Work out the finished part from the listing and answer in its coordinate system (mm). Face numbers are marked on the shaded views. A direction names the side the tool comes from. Give positions to 0.01 mm unless a question says otherwise; leave off trailing zeros. Order: outer loops, then holes, each group sorted by start corner. A loop starts at its lowest first (then second) coordinate and runs counter-clockwise, first axis right, second up.
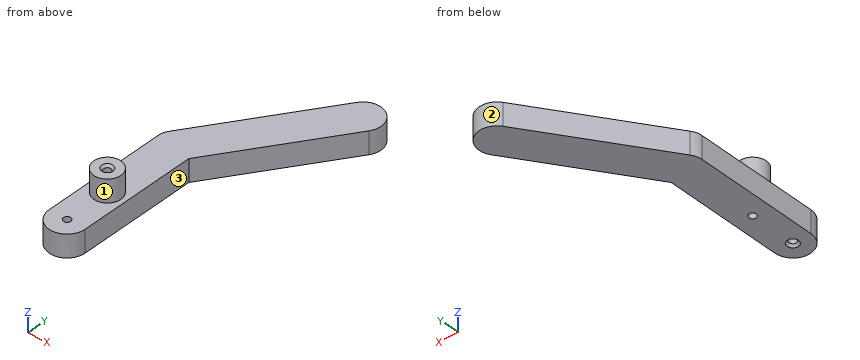
```python
from build123d import *

# Parameters (mm, degrees)
F1_DEPTH       = 6.35
F2_R           = 3.81
F3_DEPTH       = 12.7
F5_D           = 2.032
F5_CSINK_D     = 3.175
F5_CSINK_ANGLE = 82
F6_D           = 2.032
F6_CSINK_D     = 3.175
F6_CSINK_ANGLE = 82


with BuildPart() as f1:
    # F0 (on Top) → F1 (new body)
    with BuildSketch(Plane.XY):
        with BuildLine():
            ThreePointArc((-5.08, 12.7), (-3.5921024484, 9.1078975516), (0, 7.62))
            Line((0, 7.62), (0, 12.7))
            Line((0, 12.7), (0, 17.78))
            ThreePointArc((0, 17.78), (-3.5921024484, 16.2921024484), (-5.08, 12.7))
        make_face()
        with BuildLine():
            Line((0, 12.7), (0, 7.62))
            ThreePointArc((0, 7.62), (3.5921024484, 9.1078975516), (5.08, 12.7))
            ThreePointArc((5.08, 12.7), (3.5921024484, 16.2921024484), (0, 17.78))
            Line((0, 17.78), (0, 12.7))
        make_face()
        with BuildLine():
            ThreePointArc((5.08, 12.7), (3.5921024484, 9.1078975516), (0, 7.62))
            ThreePointArc((0, 7.62), (-3.5921024484, 9.1078975516), (-5.08, 12.7))
            Line((-5.08, 12.7), (-5.08, 0))
            ThreePointArc((-5.08, 0), (0, -5.08), (5.08, 0))
            Line((5.08, 0), (5.08, 12.7))
        make_face()
        with BuildLine():
            ThreePointArc((0, 17.78), (3.5921024484, 16.2921024484), (5.08, 12.7))
            Line((5.08, 12.7), (5.08, 32.7368881382))
            Line((5.08, 32.7368881382), (4.2115108686, 31.4493000504))
            ThreePointArc((4.2115108686, 31.4493000504), (2.384915539, 29.8046262283), (0, 29.21))
            Line((0, 29.21), (0, 17.78))
        make_face()
        with BuildLine():
            Line((-5.08, 34.29), (-5.08, 12.7))
            ThreePointArc((-5.08, 12.7), (-3.5921024484, 16.2921024484), (0, 17.78))
            Line((0, 17.78), (0, 29.21))
            ThreePointArc((0, 29.21), (-3.5921024484, 30.6978975516), (-5.08, 34.29))
        make_face()
        with BuildLine():
            Line((5.08, 34.29), (5.08, 32.7368881382))
            Line((5.08, 32.7368881382), (26.9371104656, 65.141386999))
            ThreePointArc((26.9371104656, 65.141386999), (25.5662995467, 72.1935978172), (18.5140887285, 70.8227868983))
            Line((18.5140887285, 70.8227868983), (-4.2115108686, 37.1306999496))
            ThreePointArc((-4.2115108686, 37.1306999496), (-0.9693096965, 39.2766660919), (2.8406999496, 38.5015108686))
            ThreePointArc((2.8406999496, 38.5015108686), (4.4853737717, 36.674915539), (5.08, 34.29))
        make_face()
        with BuildLine():
            Line((4.2115108686, 31.4493000504), (5.08, 32.7368881382))
            Line((5.08, 32.7368881382), (5.08, 34.29))
            ThreePointArc((5.08, 34.29), (4.4853737717, 36.674915539), (2.8406999496, 38.5015108686))
            Line((2.8406999496, 38.5015108686), (0, 34.29))
            Line((0, 34.29), (0, 29.21))
            ThreePointArc((0, 29.21), (2.384915539, 29.8046262283), (4.2115108686, 31.4493000504))
        make_face()
        with BuildLine():
            ThreePointArc((-4.2115108686, 37.1306999496), (-4.8580281603, 35.77524826), (-5.08, 34.29))
            ThreePointArc((-5.08, 34.29), (-3.5921024484, 30.6978975516), (0, 29.21))
            Line((0, 29.21), (0, 34.29))
            Line((0, 34.29), (2.8406999496, 38.5015108686))
            ThreePointArc((2.8406999496, 38.5015108686), (-0.9693096965, 39.2766660919), (-4.2115108686, 37.1306999496))
        make_face()
    extrude(amount=F1_DEPTH)

    # F2 (on Top) → F3 (join)
    with BuildSketch(Plane.XY):
        with Locations((0, 12.7)):
            Circle(F2_R)
    extrude(amount=F3_DEPTH)

    # F5 (through all)
    with Locations(Plane.XY.offset(12.7)):
        with Locations((0, 12.7)):
            CounterSinkHole(F5_D / 2, F5_CSINK_D / 2, counter_sink_angle=F5_CSINK_ANGLE)

    # F6 (through all)
    with Locations(Plane(origin=(0, 0, 0), x_dir=(1, 0, 0), z_dir=(0, 0, -1))):
        with Locations((0, 0)):
            CounterSinkHole(F6_D / 2, F6_CSINK_D / 2, counter_sink_angle=F6_CSINK_ANGLE)


solid = f1.part
```
1. Given P1, Ø7, axis at y = 23, z = 4, coming from the +X side; P2, Ø3, axis at y = 58.5, z = 2, coming from the +X side; P3, Ø2.5, axis at x = 0, y = 0, coming from the -Z side, each flat-ended and moving along its own axis, determine where each tip first touches the part or whether it passes through.
Findings below:
P1: stops at x = 5.08
P2: stops at x = 23.47
P3: stops at z = 0.39
2. The part is cut by section A-A (y = 12.7). Write down the section's boundary in (x, z).
Findings below:
outline: (-5.08, 0) - (-1.02, 0) - (-1.02, 12.04) - (-1.59, 12.7) - (-3.81, 12.7) - (-3.81, 6.35) - (-5.08, 6.35) - close; (1.02, 0) - (5.08, 0) - (5.08, 6.35) - (3.81, 6.35) - (3.81, 12.7) - (1.59, 12.7) - (1.02, 12.04) - close
3. Which of the six approach directions +Z, -Z, +X, -X, +Y, -Y give full straight-line access (tool end or side, diameter ignored) to the marked faces 1, 2 and 3?
Findings below:
face 1: +Z
face 2: +Z, -Z
face 3: +Z, -Z, +X, -Y
4. The part is cut by section C-C (z = 2.5). Write down the section's boundary in (x, y).
Findings below:
outline: (-5.08, 0) arc R5.08 ccw to (5.08, 0) - (5.08, 32.74) - (26.94, 65.14) arc R5.08 ccw to (18.51, 70.82) - (-4.21, 37.13) arc R5.08 ccw to (-5.08, 34.29) - close; hole circle Ø2.03 at (0, 0); hole circle Ø2.03 at (0, 12.7)
5. The part is cut by section B-B (x = 0). Write down the section's boundary in (y, z), then the cut area to 3 significant figures.
Findings below:
outline: (-5.08, 0) - (-1.59, 0) - (-1.02, 0.66) - (-1.02, 6.35) - (-5.08, 6.35) - close; (1.02, 0.66) - (1.59, 0) - (11.68, 0) - (11.68, 12.04) - (11.11, 12.7) - (8.89, 12.7) - (8.89, 6.35) - (1.02, 6.35) - close; (13.72, 0) - (43.37, 0) - (43.37, 6.35) - (16.51, 6.35) - (16.51, 12.7) - (14.29, 12.7) - (13.72, 12.04) - close
area: 317 mm2
6. Straight lines are drawn through the part: probe 1 along Y at (x, z) = (0, 2.7); probe 2 along X at (y, z) = (12.7, 9.25); probe 3 along Y at (x, z) = (0, 8.5). For each, find the intervals that lie inside material, in ascending order.
Findings below:
probe 1: y = -5.08 to -1.02, 1.02 to 11.68, 13.72 to 43.37
probe 2: x = -3.81 to -1.02, 1.02 to 3.81
probe 3: y = 8.89 to 11.68, 13.72 to 16.51
7. The part is cut by section D-D (z = 9.5). Write down the section's boundary in (x, y).
Findings below:
outline: circle Ø7.62 at (0, 12.7); hole circle Ø2.03 at (0, 12.7)
